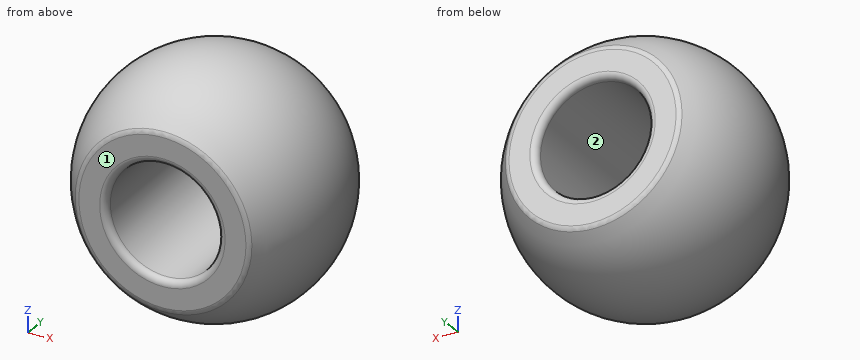
```python
from build123d import *

# Parameters (mm, degrees)
FILLET1_R = 0.3


with BuildPart() as part:
    # Sketch2 → Revolve1 (revolve)
    with BuildSketch(Plane.XY):
        with BuildLine():
            Line((2.5, -3.998088338), (2.5, 3.998088338))
            Line((2.5, 3.998088338), (3.85, 3.998088338))
            ThreePointArc((3.85, 3.998088338), (5.55042434, 0), (3.85, -3.998088338))
            Line((3.85, -3.998088338), (2.5, -3.998088338))
        make_face()
    revolve(axis=Axis((0, 0, 0), (0, 1, 0)))

    # Fillet1
    fillet1_edges = [part.edges().sort_by_distance(p)[0] for p in [
        (-3.85, 3.998088338, 0),
        (-3.85, -3.998088338, 0),
        (-2.5, -3.998088338, 0),
        (-2.5, 3.998088338, 0),
    ]]
    fillet(fillet1_edges, radius=FILLET1_R)


solid = part.part
```
Input: part model. Units: mm. Frame: model coordinates. Face numbers are marked on the shaded views. Give positions to 0.01 mm unless a question says otherwise; leave off trailing zeros. Order: outer loops, then holes, each group sorted by start corner. A loop starts at its lowest first (then second) coordinate and runs counter-clockwise, first axis right, second up. Notation, with made-up numbers: M -1,9.5 L 39,9.5 A17 ccw 39,34.5 Z; hole C 25.25,60 d5. An arc over 180 degrees is marked long. Return JSON: item names as keys, results as strings.
1) Section query A-A on y = 0.25. Output: boundary loops of the cut face in (x, z), and give its area (3 significant figures).
Taken from the geometry:
{"outline": "C 0,0 d11.09; hole C 0,0 d5", "area": "77.0 mm2"}
2) Contact query for flat-ended pins moving along their axis: pin 1 (1 mm diameter, centred on y = 1, z = -2.5, fed in from +X); pin 2 (3 mm diameter, centred on x = 2.5, y = -1, fed in from -Z); pin 3 (1 mm diameter, centred on y = -3, z = -2, fed in from +X). Output: stop coordinate, or through.
Taken from the geometry:
{"pin 1": "stops at x = 5.1", "pin 2": "stops at z = -5.42", "pin 3": "stops at x = 4.6"}
3) Section query B-B on y = -1.5. Output: boundary loops of the cut face in (x, z), and give its area (3 significant figures).
Taken from the geometry:
{"outline": "C 0,0 d10.69; hole C 0,0 d5", "area": "70.1 mm2"}
4) Mould query, pull axis X, two halves, no side actions, for the marked faces 1 and 2. Classes: released by +X, released by -X, zero draft, split by the parting line, or undercut.
Taken from the geometry:
{"face 1": "zero draft", "face 2": "undercut"}
5) Line query: L1, parallel to Z at x = 0, y = -1.5; L2, parallel to X at y = -1, z = 1; L3, parallel to Z at x = 0, y = -2. Output: solid intervals per line, ascending. Write a range as [from, to].
Taken from the geometry:
{"L1": "z = [-5.34, -2.5], [2.5, 5.34]", "L2": "x = [-5.37, -2.29], [2.29, 5.37]", "L3": "z = [-5.18, -2.5], [2.5, 5.18]"}
